from build123d import *

# Parameters (mm, degrees)
SKETCH1_R           = 25.11
SKETCH1_R_2         = 5
BOSS_EXTRUDE1_DEPTH = 2
CUT_EXTRUDE2_DEPTH  = 0.3


with BuildPart() as part:
    # Sketch1 → Boss-Extrude1 (new body)
    with BuildSketch(Plane(origin=(0, 0, 0), x_dir=(0, 0, -1), z_dir=(1, 0, 0))):
        Circle(SKETCH1_R)
        Circle(SKETCH1_R_2, mode=Mode.SUBTRACT)
    extrude(amount=BOSS_EXTRUDE1_DEPTH)

    # Sketch3 → Cut-Extrude2 (cut)
    # profile 1 of 3: a face of its own
    with BuildSketch(Plane(origin=(2, 0, 0), x_dir=(0, 0, -1), z_dir=(1, 0, 0))):
        Polygon((-21.924071507, -2.903864462), (-21.337027236, -2.903864462), (-21.337027236, -6.078864462), (-21.621963134, -6.078864462), (-21.621963134, -3.229505488), (-22.110424672, -3.229505488), align=None)
    # profile 2 of 3: a face of its own
    with BuildSketch(Plane(origin=(2, 0, 0), x_dir=(0, 0, -1), z_dir=(1, 0, 0))):
        Polygon((-18.423430481, -2.822454205), (-18.365552877, -2.822454205), (-18.365552877, -5.020531129), (-17.999206723, -5.020531129), (-17.999206723, -5.346172154), (-18.365552877, -5.346172154), (-18.365552877, -6.078864462), (-18.650488775, -6.078864462), (-18.650488775, -5.346172154), (-20.156578518, -5.346172154), align=None)
        Polygon((-18.650488775, -5.020531129), (-18.650488775, -3.641644911), (-19.596883005, -5.020531129), align=None, mode=Mode.SUBTRACT)
    # profile 3 of 3: a face of its own
    with BuildSketch(Plane(origin=(2, 0, 0), x_dir=(0, 0, -1), z_dir=(1, 0, 0))):
        Polygon((-15.981122789, -2.822454205), (-15.923245185, -2.822454205), (-15.923245185, -5.020531129), (-15.556899031, -5.020531129), (-15.556899031, -5.346172154), (-15.923245185, -5.346172154), (-15.923245185, -6.078864462), (-16.208181082, -6.078864462), (-16.208181082, -5.346172154), (-17.714270826, -5.346172154), align=None)
        Polygon((-16.208181082, -5.020531129), (-16.208181082, -3.641644911), (-17.154575313, -5.020531129), align=None, mode=Mode.SUBTRACT)
    extrude(amount=-CUT_EXTRUDE2_DEPTH, mode=Mode.SUBTRACT)


solid = part.part
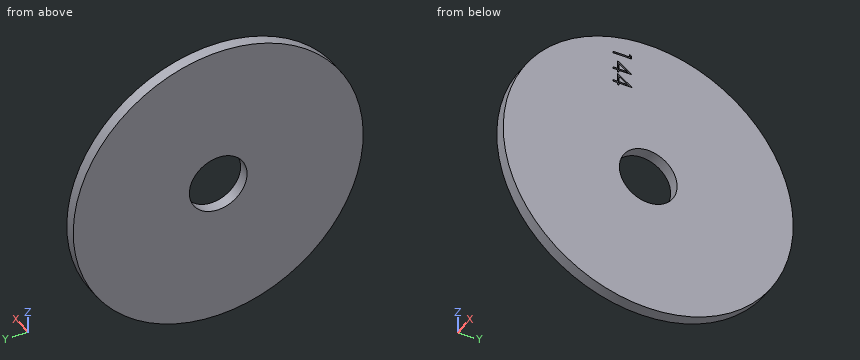
Geometry: final body of the model. Coordinates: model frame, mm. Round coordinates to 2 decimals unless told otherwise and drop trailing zeros. Loops run counter-clockwise (first coordinate to the right, second up) from the corner with the lowest first, then second, coordinate; pieces in that order, holes last. Notation, with made-up numbers: M 67.5,2 L 74.5,2 A32 cw 74.5,29 Z; hole C -30,-32 d1. An arc over 180 degrees is marked long. Put each result on its own line as item: value. Start each with the question number.
(1) Section query A-A (z = 0). Return loops of the section in (x, y).
(2) Section query C-C (x = 0.55). Return loops of the section in (y, z).
(3) Material intervals for line 1 along Y through (x, z) = (0.8, 0); line 2 along Y through (x, z) = (0.2, -1); line 3 along Z through (x, y) = (1.95, 5.5), sorted ascending. Write a range as [from, to].
(4) Section query D-D (y = 12). Return loops of the section in (x, z), then the cut area to 3 significant figures.
Findings below:
1. outline: M 0,-25.11 L 2,-25.11 L 2,-5 L 0,-5 Z; M 0,5 L 2,5 L 2,25.11 L 0,25.11 Z
2. outline: C 0,0 d50.22; hole C 0,0 d10
3. line 1: y = [-25.11, -5], [5, 25.11]
3. line 2: y = [-25.09, -4.9], [4.9, 25.09]
3. line 3: z = [-24.5, 24.5]
4. outline: M 0,-22.06 L 2,-22.06 L 2,22.06 L 0,22.06 Z
4. area: 88.2 mm2
